Autodesk Inventor part; units mm, degrees
ref_plane "YZ Plane" through (0, 0, 0) normal (1, 0, 0) x (0, 1, 0)
ref_plane "XZ Plane" through (0, 0, 0) normal (0, 1, 0) x (-1, 0, 0)
ref_plane "XY Plane" through (0, 0, 0) normal (0, 0, 1) x (1, 0, 0)
sketch "Sketch1" plane through (0, 0, 0) normal (1, 0, 0) x (0, 1, 0)
  circle A0 centre (0, 0) radius 129
  circle A1 centre (0, 0) radius 125.5
  dimension "d0" = 258
  dimension "d1" = 251
extrude "Extrusion1" add sketch "Sketch1" along normal blind 80
sketch "Sketch2" plane through (80, 0, 0) normal (1, 0, 0) x (0, 0, -1)
  line L0 (-101.4747, 92.723) -> (-414.8501, 828.7908)
  line L1 (-414.8501, 828.7908) -> (195.4959, 828.7908)
  line L2 (195.4959, 828.7908) -> (66.4648, 110.5596)
  circle A0 centre (0, 0) radius 129
  line L3 (-101.4747, 92.723) -> (-97.8081, 84.1106)
  line L4 (118.8614, 50.1294) -> (856.9556, 272.0827)
  line L5 (856.9556, 272.0827) -> (856.9556, -315.7415)
  line L6 (856.9556, -315.7415) -> (112.0393, -63.9391)
  line L7 (-127.8547, 17.1518) -> (-838.6795, -370.3737)
  line L8 (-838.6795, -370.3737) -> (-437.3695, -726.566)
  line L9 (-437.3695, -726.566) -> (-54.85, -116.7582)
  dimension "d4" = 800
extrude "Extrusion2" add sketch "Sketch2" against normal blind 80 contours L0 L1 L2 A0 L3 | A0 L9 L8 L7 | L4 L5 L6 A0
properties part number "fan blade"
For this review, take the finished solid that the model builds, in its own axes (mm). A direction names the side the tool comes from. Round coordinates to 2 decimals unless told otherwise and drop trailing zeros. Loops run counter-clockwise (first coordinate to the right, second up) from the corner with the lowest first, then second, coordinate; pieces in that order, holes last. Notation, with made-up numbers: (9, -26.75) - (56, -26.75) arc R35 ccw to (56, 7.25) - close; hole circle Ø4 at (23, 36). An arc over 180 degrees is marked (long way). One line per item, written item: value. Start each with the question number.
Item 1: The part is to be moulded in two halves that separate along Y. For faces 6 (the flat face through (41, 828.791, 114)), 7 (the cylindrical face through (39.44, 52.337, 117.906)), 8 (the cylindrical face through (39.44, 84.94, -97.09)), 9 (the cylindrical face through (39.44, -122.574, -40.206)), say which applies: +Y half, -Y half, draft (parallel to the pull), parting line (faces both ways), or undercut.
Item 2: Clearance check with flat-ended pins moving along their axes: pin 1 Ø12 at (x, z) = (59.5, -618) entering from +Y; pin 2 Ø8 at (x, z) = (62.5, 647.5) entering from -Y; pin 3 Ø4 at (x, z) = (35.5, -623) entering from -Y. State where each tip first meets the part, or that it passes through.
Item 3: Take a section at D-D (y = 356.5). Give the boundary of the cut face in (x, z), plus the area to 3 significant figures.
Item 4: For L1, parallel to Y at x = 10, z = -30.5; L2, parallel to Z at x = 37, y = 0; L3, parallel to Y at x = 65, z = 379, list the stretches that pass through material, from the lowest coordinate up.
Item 5: Take a section at C-C (x = 33.5). Give the boundary of the cut face in (y, z).
Item 6: For faces 1 (the flat face through (40.56, -173.898, 478.291)), 2 (the flat face through (40.6, -191.6, -489.7)), 3 (the flat face through (40.56, 474.703, -131.884)), 4 (the flat face through (0, 163, -68)), 5 (the flat face through (41, -18, -856.956)), list the 3-axis set-ups (+Z, -Z, +X, -X, +Y, -Y) from which the entire face can be reached by the end or side of a thin tool; tool diameter is ignored.
Item 7: Take a section at A-A (z = 0). Give the boundary of the cut face in (x, y).
Item 8: Take a section at B-B (y = -197). Give the boundary of the cut face in (x, z).
Answer below:
1. face 6: +Y half
1. face 7: undercut
1. face 8: undercut
1. face 9: -Y half
2. pin 1: stops at y = 202.03
2. pin 2: stops at y = -543.61
2. pin 3: stops at y = -237.33
3. outline: (0, -110.65) - (80, -110.65) - (80, 213.78) - (0, 213.78) - close
3. area: 26,000 mm2
4. L1: y = -125.34 to -121.74, 121.74 to 828.79
4. L2: z = -856.96 to -125.5, 125.5 to 159.32
4. L3: y = -633.51 to -119.77, 744.58 to 828.79
5. outline: (-726.57, 437.37) - (-116.76, 54.85) arc R129 ccw to (-63.94, -112.04) - (-315.74, -856.96) - (272.08, -856.96) - (50.13, -118.86) arc R129 ccw to (110.56, -66.46) - (828.79, -195.5) - (828.79, 414.85) - (92.72, 101.47) - (84.11, 97.81) arc R129 ccw to (17.15, 127.85) - (-370.37, 838.68) - close; hole circle Ø251 at (0, 0)
6. face 1: +Z, +X, -X
6. face 2: +X, -X, -Y
6. face 3: +X, -X
6. face 4: +Z, -Z, -X, +Y, -Y
6. face 5: -Z, +X, -X, +Y, -Y
7. outline: (0, -129) - (80, -129) - (80, -125.5) - (0, -125.5) - close; (0, 125.5) - (80, 125.5) - (80, 828.79) - (0, 828.79) - close
8. outline: (0, -856.96) - (80, -856.96) - (80, -505.68) - (0, -505.68) - close; (0, 105.18) - (80, 105.18) - (80, 520.67) - (0, 520.67) - close
